Could you check a few things on this model? Use its own coordinates, in mm. A direction names the side the tool comes from. Round coordinates to 2 decimals unless told otherwise and drop trailing zeros. Write each question's results on one line, items separated by ' | '. Start each with the question number.
1) We'd pull the mould along Z, two halves only. Please class faces 3 (the flat face through (41, 7, 0)), 4 (the flat face through (-1, 7, 25)), 5 (the conical face through (-18.1, 5.08, 12.26)): pulls with the +Z half, pulls with the -Z half, needs draft (parallel to the pull), parting line crosses it, or undercut.
2) Which directions (+Z, -Z, +X, -X, +Y, -Y) give clear straight access to the entire face, cutting with the end or side of a thin tool? Please do faces 1 (the flat face through (-0.6, 15.3, -24.2)), 2 (the cylindrical face through (21.06, 6.94, 13.5)).
3) If I drill on probe 1 along X at (y, z) = (7.55, 12.5); probe 2 along Z at (x, y) = (-18.25, 7.2); probe 3 along X at (y, z) = (12.5, 12.5), over which ranges is the centre line in solid material (lowest first)?
4) For P1, Ø2, axis at x = 19.75, z = 12.5, coming from the -Y side; P2, Ø2, axis at x = -18.5, z = -12.5, coming from the +Y side; P3, Ø3, axis at x = 19.5, z = 12.5, coming from the +Y side; P4, Ø3, axis at x = 19.75, z = 12.5, coming from the +Y side, each with a flat end and sliding along its axis, tell me the tip position at first contact or that it passes through.
from build123d import *

# Parameters (mm, degrees)
SKETCH1_W                   = 82
SKETCH1_H                   = 50
BOSS_EXTRUDE1_DEPTH         = 16
CHAMFER1_SIZE               = 1.5
M4_TAPPED_HOLE3_D           = 3.3
M4_TAPPED_HOLE3_DEPTH       = 10.1
M4_TAPPED_HOLE3_CBORE_D     = 4
M4_TAPPED_HOLE3_CBORE_DEPTH = 8
M4_TAPPED_HOLE3_TIP         = 0.991420021


with BuildPart() as part:
    # Sketch1 → Boss-Extrude1 (new body)
    with BuildSketch(Plane(origin=(0, 0, 0), x_dir=(1, 0, 0), z_dir=(0, 1, 0))):
        Rectangle(SKETCH1_W, SKETCH1_H)
    extrude(amount=BOSS_EXTRUDE1_DEPTH)

    # Chamfer1
    chamfer1_edges = [part.edges().sort_by_distance(p)[0] for p in [
        (41, 16, 0),
        (0, 16, -25),
        (-41, 16, 0),
        (0, 16, 25),
    ]]
    chamfer(chamfer1_edges, length=CHAMFER1_SIZE)

    # M4 Tapped Hole3
    with Locations(Plane(origin=(0, 16, 0), x_dir=(1, 0, 0), z_dir=(0, 1, 0))):
        with Locations((-18.25, -12.5), (19.75, 12.5), (-18.25, 12.5), (19.75, -12.5)):
            CounterBoreHole(M4_TAPPED_HOLE3_D / 2, M4_TAPPED_HOLE3_CBORE_D / 2, M4_TAPPED_HOLE3_CBORE_DEPTH, depth=M4_TAPPED_HOLE3_DEPTH)
            with Locations((0, 0, -(M4_TAPPED_HOLE3_DEPTH + M4_TAPPED_HOLE3_TIP / 2))):  # 118° drill point
                Cone(0, M4_TAPPED_HOLE3_D / 2, M4_TAPPED_HOLE3_TIP, mode=Mode.SUBTRACT)


solid = part.part
Checked values:
1) face 3: needs draft | face 4: pulls with the +Z half | face 5: undercut
2) face 1: -Z, +X, -X, +Y | face 2: +Y
3) probe 1: -41 to -19.9, -16.6 to 18.1, 21.4 to 41 | probe 2: -25 to -14.15, -10.85 to 10.85, 14.15 to 25 | probe 3: -41 to -20.25, -16.25 to 17.75, 21.75 to 41
4) P1: y = 0 | P2: y = 5.66 | P3: y = 8 | P4: y = 5.81
